The listing builds one solid part. Answer for the finished solid, in the listing's coordinates (mm). Face numbers are marked on the shaded views. A direction names the side the tool comes from. Give positions to 0.01 mm unless a question says otherwise; leave off trailing zeros. Order: outer loops, then holes, each group sorted by start corner. A loop starts at its lowest first (then second) coordinate and runs counter-clockwise, first axis right, second up. Notation, with made-up numbers: (87.25, 81) - (142.25, 81) arc R19 ccw to (142.25, 93) - close; hole circle Ø3 at (81.5, 85.25). An arc over 180 degrees is marked (long way). Answer in a Markdown table with one row per item. Add a question column.
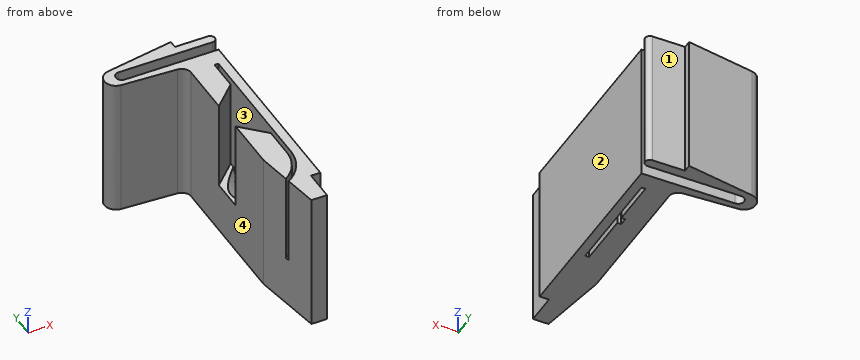
```python
from build123d import *

# Parameters (mm, degrees)
PAD006_DEPTH    = 18
POCKET004_DEPTH = 18
POCKET005_DEPTH = 18


with BuildPart() as part:
    # Sketch010 → Pad006 (new body)
    with BuildSketch(Plane.XY):
        with BuildLine():
            Line((178, 0), (176, 0))
            Line((176, 0), (174.5, 9))
            Line((174.5, 27), (174.5, 9))
            ThreePointArc((174.5, 27), (174.171415, 27.825006), (173.365608, 28.198205))
            Line((173.365608, 28.198205), (166.36958, 28.581273))
            ThreePointArc((166.202763, 31.5), (164.98147, 29.966068), (166.36958, 28.581273))
            Line((175, 33), (166.202763, 31.5))
            Line((175, 33), (175, 32))
            Line((175, 32), (179.2, 32))
            ThreePointArc((179.2, 30.8), (179.8, 31.4), (179.2, 32))
            Line((179.2, 30.8), (167.2, 30.8))
            ThreePointArc((167.2, 30.8), (166.45, 30.05), (167.2, 29.3))
            Line((179.2, 29.3), (167.2, 29.3))
            Line((179.2, 29.3), (179.2, 4))
            Line((179.2, 4), (178, 4))
            Line((178, 4), (178, 0))
        make_face()
    extrude(amount=PAD006_DEPTH)

    # Sketch011 → Groove001 (revolve, cut)
    with BuildSketch(Plane.XY.offset(9)):
        Polygon((174.2, 18), (174.2, 19.8), (177.5, 23), (177.5, 27), (178, 27), (178, 18), align=None)
    revolve(axis=Axis((0, 18, 9), (-1, 0, 0)), mode=Mode.SUBTRACT)

    # Sketch012 → Pocket004 (cut)
    with BuildSketch(Plane.XY.offset(6.5)):
        with BuildLine():
            Line((178, 27), (177.5, 27))
            Line((177.5, 27), (177.5, 23))
            Line((177.5, 23), (174.2, 19.8))
            Line((174.2, 19.8), (174.2, 16.2))
            Line((174.2, 16.2), (177.5, 13))
            Line((177.5, 13), (177.5, 9))
            ThreePointArc((172.5, 4), (176.035534, 5.464466), (177.5, 9))
            Line((172.5, 4), (172.5, 3.5))
            ThreePointArc((172.5, 3.5), (176.389087, 5.110913), (178, 9))
            Line((178, 9), (178, 27))
        make_face()
    extrude(amount=POCKET004_DEPTH, mode=Mode.SUBTRACT)

    # Sketch013 → Pocket005 (cut)
    with BuildSketch(Plane.XY):
        Polygon((177.5, 27), (178, 27), (178, 13), (177.5, 13), (177.5, 20), (177, 20), (177, 21), (177.5, 21), align=None)
    extrude(amount=POCKET005_DEPTH, mode=Mode.SUBTRACT)


solid = part.part
```
(1) For the marked faces 1, 2, 3 and 4, determine the directions among +Z, -Z, +X, -X, +Y, -Y from which every point of the face is accessible in a straight line to the end or side of a thin tool.
(2) Find section B-B, the plane z = 12.5. Write down the section's boundary in (x, y).
(3) Find section C-C, the plane y = 12. Write down the section's boundary in (x, z), plus the area to 3 significant figures.
(4) Each of these flat-tipped pins is pushed along its axis until it touches: P1, Ø1.5, axis at x = 175.5, y = 19, coming from the +Z side; P2, Ø0.6, axis at x = 179, z = 6.5, coming from the -Y side; P3, Ø3.5, axis at x = 171, z = 9.5, coming from the -Y side. Where does it stop, or does it pass through?
(5) Find section D-D, the plane x = 169.25. Write down the section's boundary in (y, z), plus the area to 3 significant figures.
(6) Find section A-A, the plane x = 178.75. Write down the section's boundary in (y, z).
(7) Straight lines are drawn through the part: line 1 (Y direction, x = 175.25, z = 11); line 2 (Y direction, x = 176.75, z = 13.75); line 3 (X direction, y = 12.5, z = 12.25). For each, find the intervals that lie inside material, in ascending order.
Answer key:
| question | item | result |
|---|---|---|
| 1 | face 1 | +Z, -Z, +X, +Y |
| 1 | face 2 | +Z, -Z, +X, -Y |
| 1 | face 3 | +Z |
| 1 | face 4 | +Z, -Z, -X, -Y |
| 2 | outline | (166.2, 31.5) arc R1.47 ccw to (166.37, 28.58) - (173.37, 28.2) arc R1.2 cw to (174.5, 27) - (174.5, 20.09) - (177.5, 23) - (177.5, 27) - (178, 27) - (178, 9) arc R5.5 cw to (175.29, 4.26) - (176, 0) - (178, 0) - (178, 4) - (179.2, 4) - (179.2, 29.3) - (167.2, 29.3) arc R0.75 cw to (167.2, 30.8) - (179.2, 30.8) arc R0.6 ccw to (179.2, 32) - (175, 32) - (175, 33) - close; (174.5, 9) - (175.2, 4.79) arc R5 ccw to (177.5, 9) - (177.5, 13) - (174.5, 15.91) - close |
| 3 | outline | (174.5, 0) - (179.2, 0) - (179.2, 18) - (178, 18) - (178, 2.29) - (177.5, 2.29) - (177.5, 18) - (174.5, 18) - close |
| 3 | area | 76.7 mm² |
| 4 | P1 | z = 6.5 |
| 4 | P2 | y = 4 |
| 4 | P3 | y = 28.23 |
| 5 | outline | (28.42, 0) - (29.3, 0) - (29.3, 18) - (28.42, 18) - close; (30.8, 0) - (32.02, 0) - (32.02, 18) - (30.8, 18) - close |
| 5 | area | 37.7 mm² |
| 6 | outline | (4, 0) - (29.3, 0) - (29.3, 18) - (4, 18) - close; (30.8, 0) - (32, 0) - (32, 18) - (30.8, 18) - close |
| 7 | line 1 | 4.82 to 15.18, 20.82 to 29.3, 30.8 to 32 |
| 7 | line 2 | 0 to 5.51, 6.37 to 13.73, 22.27 to 29.3, 30.8 to 32 |
| 7 | line 3 | 174.5 to 177.5, 178 to 179.2 |
